Read the model definition and answer for the solid it produces. Units are mm, in the model's axes. A direction names the side the tool comes from. Give positions to 0.01 mm unless a question says otherwise; leave off trailing zeros. Write each loop counter-clockwise with the first axis right and the second up, starting at its lowest first coordinate (ties: lowest second). Pieces come first, ordered by that corner, then holes. Notation, with made-up numbers: M 14.5,74.5 L 27.5,74.5 A14 cw 27.5,88.5 Z; hole C 84.25,20 d8. An arc over 180 degrees is marked long. Write each question's results on one line, items separated by ' | '. Start each with the question number.
```python
from build123d import *

# Parameters (mm, degrees)
ESQUISSE1_R        = 15
BOSS_EXTRU_1_DEPTH = 10


with BuildPart() as part:
    # Esquisse1 → Boss.-Extru.1 (new body)
    with BuildSketch(Plane.XY):
        with BuildLine():
            Line((-38.97114317, 22.5), (43.202021157, 164.828095634))
            Line((43.202021157, 164.828095634), (43.202021157, 12.59306825))
            Line((43.202021157, 12.59306825), (143.202021157, 131.768427509))
            Line((143.202021157, 131.768427509), (143.202021157, 100.653950972))
            Line((143.202021157, 100.653950972), (34.47199994, -28.925442436))
            ThreePointArc((34.47199994, -28.925442436), (-25.810939636, -36.861841993), (-38.97114317, 22.5))
        make_face()
        Circle(ESQUISSE1_R, mode=Mode.SUBTRACT)
    extrude(amount=BOSS_EXTRU_1_DEPTH)


solid = part.part
```
Item 1: For faces 1 (the flat face through (1.54, 92.67, 4.93)), 2 (the flat face through (43.202, 90, 5)), determine the directions among +Z, -Z, +X, -X, +Y, -Y from which every point of the face is accessible in a straight line to the end or side of a thin tool.
Item 2: Determine the mould class of faces 3 (the flat face through (89.598, 36.771, 4.93)), 4 (the cylindrical face through (-25.04, -37.39, 4.93)), 5 (the cylindrical face through (-14.985, 0.66, 4.93)), 6 (the flat face through (143.202, 116, 5)) for opening direction Y: +Y half, -Y half, draft (parallel to the pull), parting line (faces both ways), or undercut.
Item 3: Section D-D, the plane x = 78.5 is taken. Determine the outline of the cut face in (y, z), then the cut area to 3 significant figures.
Item 4: Section C-C, the plane y = 8.5 is taken. Determine the outline of the cut face in (x, z), then the cut area to 3 significant figures.
Item 5: Straight lines are drawn through the part: line 1 (Y direction, x = 0, z = 6.75); line 2 (X direction, y = 124.5, z = 5); line 3 (X direction, y = -7.5, z = 2). For each, find the intervals that lie inside material, in ascending order.
Item 6: Section A-A, the plane x = 0 is taken. Determine the outline of the cut face in (y, z), then the cut area to 3 significant figures.
Item 7: Section B-B, the plane z = 4 is taken. Determine the outline of the cut face in (x, y).
Item 8: Given P1, Ø4, axis at x = 32.5, z = 3, coming from the +Y side; P2, Ø1.5, axis at x = 50.5, z = 2.5, coming from the -Y side; P3, Ø5, axis at y = 55, z = 4.5, coming from the +X side; P4, Ø18, axis at x = 0, y = 0, coming from the +Z side, each flat-ended and moving along its own axis, determine where each tip first touches the part or whether it passes through.
Worked out:
1) face 1: +Z, -Z, -X, +Y | face 2: +Z, -Z, +Y
2) face 3: -Y half | face 4: parting line | face 5: undercut | face 6: draft
3) outline: M 23.55,0 L 54.66,0 L 54.66,10 L 23.55,10 Z | area: 311 mm²
4) outline: M -44.19,0 L -12.36,0 L -12.36,10 L -44.19,10 Z; M 12.36,0 L 65.88,0 L 65.88,10 L 12.36,10 Z | area: 853 mm²
5) line 1: y = -45 to -15, 15 to 90 | line 2: x = 19.92 to 43.2, 137.1 to 143.2 | line 3: x = -44.37 to -12.99, 12.99 to 52.45
6) outline: M -45,0 L -15,0 L -15,10 L -45,10 Z; M 15,0 L 90,0 L 90,10 L 15,10 Z | area: 1,050 mm²
7) outline: M -38.97,22.5 A45 ccw 34.47,-28.93 L 143.2,100.65 L 143.2,131.77 L 43.2,12.59 L 43.2,164.83 Z; hole C 0,0 d30
8) P1: stops at y = 149.76 | P2: stops at y = -10.72 | P3: stops at x = 106.99 | P4: passes through
